from build123d import *
from build123d.topology import SkipClean

# Parameters (mm, degrees)
SKETCH_1_W          = 86
SKETCH_1_H          = 68
SKETCH_1_R          = 1.8
EXTRUDE_1_DEPTH     = 3
CUT_EXTRUDE_1_DEPTH = 3
SKETCH_3_W          = 30
SKETCH_3_H          = 6
SKETCH_3_R          = 1.6
EXTRUDE_2_DEPTH     = 3
EXTRUDE_3_DEPTH     = 3
SKETCH_5_R          = 1.5
CUT_EXTRUDE_2_DEPTH = 79.276480437
CUT_EXTRUDE_3_DEPTH = 79.276480437
EXTRUDE_4_DEPTH     = 3
EXTRUDE_6_DEPTH     = 3
CUT_EXTRUDE_6_DEPTH = 85.85098703
CUT_EXTRUDE_7_DEPTH = 85.85098703


with BuildPart() as part:
    # 草图1 → 凸台-拉伸1 (new body)
    with BuildSketch(Plane(origin=(0, 0, 0), x_dir=(1, 0, 0), z_dir=(0, 1, 0))):
        Rectangle(SKETCH_1_W, SKETCH_1_H)
        with Locations(Location((-36, -27, 0), (0, 0, 270))):
            Circle(SKETCH_1_R, mode=Mode.SUBTRACT)
        with Locations(Location((-36, 27, 0), (0, 0, 270))):
            Circle(SKETCH_1_R, mode=Mode.SUBTRACT)
        with Locations(Location((36, 27, 0), (0, 0, 270))):
            Circle(SKETCH_1_R, mode=Mode.SUBTRACT)
        with Locations(Location((36, -27, 0), (0, 0, 270))):
            Circle(SKETCH_1_R, mode=Mode.SUBTRACT)
    extrude(amount=EXTRUDE_1_DEPTH)

    # 草图2 → 切除-拉伸1 (cut)
    with BuildSketch(Plane.XZ):
        Polygon((26, 25), (35, 34), (-35, 34), (-26, 25), align=None)
        Polygon((-28, 13), (-43, 28), (-43, -28), (-28, -13), align=None)
        Polygon((-35, -34), (35, -34), (26, -25), (-26, -25), align=None)
        Polygon((43, -28), (43, 28), (28, 13), (28, -13), align=None)
    extrude(amount=-CUT_EXTRUDE_1_DEPTH, mode=Mode.SUBTRACT)

    # 草图3 → 凸台-拉伸2 (add)
    # profile 1 of 3: a face of its own
    with BuildSketch(Plane.XZ):
        Polygon((35, 34), (43, 34), (45.67228251, 57.499999999), (15.67228251, 57.499999999), (26, 25), align=None)
    # profile 2 of 3: a face of its own
    with BuildSketch(Plane.XZ):
        with Locations((30.67228251, 60.499999999)):
            Rectangle(SKETCH_3_W, SKETCH_3_H)
        with Locations(Location((20.67228251, 60.499999999, 0), (0, 0, 270))):
            Circle(SKETCH_3_R, mode=Mode.SUBTRACT)
        with Locations(Location((40.67228251, 60.499999999, 0), (0, 0, 270))):
            Circle(SKETCH_3_R, mode=Mode.SUBTRACT)
    # profile 3 of 3: a face of its own
    with BuildSketch(Plane.XZ):
        Polygon((45.67228251, -63.499999999), (45.67228251, -57.499999999), (43, -34), (35, -34), (26, -25), (15.67228251, -57.499999999), (15.67228251, -63.499999999), align=None)
        with Locations(Location((20.67228251, -60.499999999, 0), (0, 0, 270))):
            Circle(SKETCH_3_R, mode=Mode.SUBTRACT)
        with Locations(Location((40.67228251, -60.499999999, 0), (0, 0, 270))):
            Circle(SKETCH_3_R, mode=Mode.SUBTRACT)
    extrude(amount=-EXTRUDE_2_DEPTH)

    # 草图4 → 凸台-拉伸3 (add)
    with BuildSketch(Plane.XZ):
        Polygon((15.67228251, 57.499999999), (15.67228251, 63.499999999), (-43, 34), (-35, 34), align=None)
        Polygon((-35, -34), (-43, -34), (15.67228251, -63.499999999), (15.67228251, -57.499999999), align=None)
    extrude(amount=-EXTRUDE_3_DEPTH)

    # 草图5 → 切除-拉伸2 (cut, through all)
    with BuildSketch(Plane.XZ):
        with Locations(Location((-13.9, 10, 0), (0, 0, 270))):
            Circle(SKETCH_5_R)
        with Locations(Location((14.8, 10, 0), (0, 0, 270))):
            Circle(SKETCH_5_R)
        with Locations(Location((-13.9, -10, 0), (0, 0, 270))):
            Circle(SKETCH_5_R)
        with Locations(Location((14.8, -10, 0), (0, 0, 270))):
            Circle(SKETCH_5_R)
    extrude(amount=-CUT_EXTRUDE_2_DEPTH, mode=Mode.SUBTRACT)

    # 草图6 → 切除-拉伸3 (cut, through all)
    with BuildSketch(Plane.XZ):
        with BuildLine():
            Line((-21.292893219, 20.292893219), (-14.292893219, 13.292893219))
            ThreePointArc((-14.292893219, 13.292893219), (-13.96846987, 13.076120467), (-13.585786438, 13))
            Line((-13.585786438, 13), (13.485786438, 13))
            ThreePointArc((13.485786438, 13), (13.86846987, 13.076120467), (14.192893219, 13.292893219))
            Line((14.192893219, 13.292893219), (21.192893219, 20.292893219))
            ThreePointArc((21.192893219, 20.292893219), (21.40966597, 21.382683432), (20.485786438, 22))
            Line((20.485786438, 22), (-20.585786438, 22))
            ThreePointArc((-20.585786438, 22), (-21.50966597, 21.382683432), (-21.292893219, 20.292893219))
        make_face()
        with BuildLine():
            Line((-25, 7.585786438), (-25, -7.585786438))
            ThreePointArc((-25, -7.585786438), (-24.382683432, -8.50966597), (-23.292893219, -8.292893219))
            Line((-23.292893219, -8.292893219), (-17.192893219, -2.192893219))
            ThreePointArc((-17.192893219, -2.192893219), (-16.976120467, -1.86846987), (-16.9, -1.485786438))
            Line((-16.9, -1.485786438), (-16.9, 1.485786438))
            ThreePointArc((-16.9, 1.485786438), (-16.976120467, 1.86846987), (-17.192893219, 2.192893219))
            Line((-17.192893219, 2.192893219), (-23.292893219, 8.292893219))
            ThreePointArc((-23.292893219, 8.292893219), (-24.382683432, 8.50966597), (-25, 7.585786438))
        make_face()
        with BuildLine():
            Line((-9.9, 9), (9.9, 9))
            ThreePointArc((9.9, 9), (10.607106781, 8.707106781), (10.9, 8))
            Line((10.9, 8), (10.9, -8))
            ThreePointArc((10.9, -8), (10.607106781, -8.707106781), (9.9, -9))
            Line((9.9, -9), (-9.9, -9))
            ThreePointArc((-9.9, -9), (-10.607106781, -8.707106781), (-10.9, -8))
            Line((-10.9, -8), (-10.9, 8))
            ThreePointArc((-10.9, 8), (-10.607106781, 8.707106781), (-9.9, 9))
        make_face()
        with BuildLine():
            Line((14.192893219, -13.292893219), (21.192893219, -20.292893219))
            ThreePointArc((21.192893219, -20.292893219), (21.40966597, -21.382683432), (20.485786438, -22))
            Line((20.485786438, -22), (-20.585786438, -22))
            ThreePointArc((-20.585786438, -22), (-21.50966597, -21.382683432), (-21.292893219, -20.292893219))
            Line((-21.292893219, -20.292893219), (-14.292893219, -13.292893219))
            ThreePointArc((-14.292893219, -13.292893219), (-13.96846987, -13.076120467), (-13.585786438, -13))
            Line((-13.585786438, -13), (13.485786438, -13))
            ThreePointArc((13.485786438, -13), (13.86846987, -13.076120467), (14.192893219, -13.292893219))
        make_face()
        with BuildLine():
            Line((16.9, -1.485786438), (16.9, 1.485786438))
            ThreePointArc((16.9, 1.485786438), (16.976120467, 1.86846987), (17.192893219, 2.192893219))
            Line((17.192893219, 2.192893219), (23.292893219, 8.292893219))
            ThreePointArc((23.292893219, 8.292893219), (24.382683432, 8.50966597), (25, 7.585786438))
            Line((25, 7.585786438), (25, -7.585786438))
            ThreePointArc((25, -7.585786438), (24.382683432, -8.50966597), (23.292893219, -8.292893219))
            Line((23.292893219, -8.292893219), (17.192893219, -2.192893219))
            ThreePointArc((17.192893219, -2.192893219), (16.976120467, -1.86846987), (16.9, -1.485786438))
        make_face()
    extrude(amount=-CUT_EXTRUDE_3_DEPTH, mode=Mode.SUBTRACT)

    # 草图7 → 凸台-拉伸4 (add)
    with BuildSketch(Plane.XZ):
        Polygon((-56.2, 27.363135311), (-56.2, -27.363135311), (-43, -34), (-43, -28), (-52.2, -23.374306429), (-52.2, 23.374306429), (-43, 28), (-43, 34), align=None)
    extrude(amount=-EXTRUDE_4_DEPTH)

    # 草图11 → 凸台-拉伸6 (add)
    with BuildSketch(Plane.XZ):
        with BuildLine():
            Line((35.3, 1.5), (35.3, 18.5))
            ThreePointArc((35.3, 18.5), (34.629179607, 18.658359214), (34.1, 19.1))
            Line((34.1, 19.1), (28, 13))
            Line((28, 13), (28, -13))
            Line((28, -13), (34.1, -19.1))
            ThreePointArc((34.1, -19.1), (34.629179607, -18.658359214), (35.3, -18.5))
            Line((35.3, -18.5), (35.3, -1.5))
            ThreePointArc((35.3, -1.5), (33.8, 0), (35.3, 1.5))
        make_face()
        with BuildLine():
            ThreePointArc((36.8, 20), (36.360660172, 18.939339828), (35.3, 18.5))
            Line((35.3, 18.5), (35.3, 1.5))
            ThreePointArc((35.3, 1.5), (36.360660172, 1.060660172), (36.8, 0))
            ThreePointArc((36.8, 0), (36.360660172, -1.060660172), (35.3, -1.5))
            Line((35.3, -1.5), (35.3, -18.5))
            ThreePointArc((35.3, -18.5), (36.360660172, -18.939339828), (36.8, -20))
            ThreePointArc((36.8, -20), (36.641640786, -20.670820393), (36.2, -21.2))
            Line((36.2, -21.2), (38.3, -23.3))
            Line((38.3, -23.3), (38.3, 23.3))
            Line((38.3, 23.3), (36.2, 21.2))
            ThreePointArc((36.2, 21.2), (36.641640786, 20.670820393), (36.8, 20))
        make_face()
    extrude(amount=-EXTRUDE_6_DEPTH)

    # 草图11<3> → 切除-拉伸6 (cut, through all)
    with SkipClean():  # the faces are left unmerged after this step: merging them gives an invalid solid
        with BuildSketch(Plane.XZ):
            with BuildLine():
                ThreePointArc((36.2, 21.2), (34.239339828, 21.060660172), (34.1, 19.1))
                Line((34.1, 19.1), (36.2, 21.2))
            make_face()
            with BuildLine():
                Line((36.2, 21.2), (34.1, 19.1))
                ThreePointArc((34.1, 19.1), (35.774341649, 18.576975053), (36.8, 20))
                ThreePointArc((36.8, 20), (36.641640786, 20.670820393), (36.2, 21.2))
            make_face()
            with BuildLine():
                ThreePointArc((36.8, -20), (35.774341649, -18.576975053), (34.1, -19.1))
                Line((34.1, -19.1), (36.2, -21.2))
                ThreePointArc((36.2, -21.2), (36.641640786, -20.670820393), (36.8, -20))
            make_face()
            with BuildLine():
                Line((36.2, -21.2), (34.1, -19.1))
                ThreePointArc((34.1, -19.1), (34.239339828, -21.060660172), (36.2, -21.2))
            make_face()
        extrude(amount=-CUT_EXTRUDE_6_DEPTH, mode=Mode.SUBTRACT)

    # 草图12 → 切除-拉伸7 (cut, through all)
    with SkipClean():  # the faces are left unmerged after this step: merging them gives an invalid solid
        with BuildSketch(Plane.XZ):
            with BuildLine():
                Line((21.125963718, 53.545721451), (27.85115527, 32.382407713))
                ThreePointArc((27.85115527, 32.382407713), (29.426324108, 31.343770669), (30.771106367, 32.667207276))
                Line((30.771106367, 32.667207276), (33.177674586, 53.830521014))
                ThreePointArc((33.177674586, 53.830521014), (32.806256586, 54.998944823), (31.687279714, 55.499999999))
                Line((31.687279714, 55.499999999), (22.555519943, 55.499999999))
                ThreePointArc((22.555519943, 55.499999999), (21.344855286, 54.885602104), (21.125963718, 53.545721451))
            make_face()
            with BuildLine():
                Line((30.771106367, -32.667207276), (33.177674586, -53.830521014))
                ThreePointArc((33.177674586, -53.830521014), (32.806256586, -54.998944823), (31.687279714, -55.499999999))
                Line((31.687279714, -55.499999999), (22.555519943, -55.499999999))
                ThreePointArc((22.555519943, -55.499999999), (21.344855286, -54.885602104), (21.125963718, -53.545721451))
                Line((21.125963718, -53.545721451), (27.85115527, -32.382407713))
                ThreePointArc((27.85115527, -32.382407713), (29.426324108, -31.343770669), (30.771106367, -32.667207276))
            make_face()
        extrude(amount=-CUT_EXTRUDE_7_DEPTH, mode=Mode.SUBTRACT)


solid = part.part
Read the model definition and answer for the solid it produces. Units are mm, in the model's axes. Give positions to 0.01 mm unless a question says otherwise; leave off trailing zeros. Write each loop counter-clockwise with the first axis right and the second up, starting at its lowest first coordinate (ties: lowest second). Pieces come first, ordered by that corner, then holes. Notation, with made-up numbers: M -37.5,39.25 L 10.5,39.25 A18 cw 10.5,53.25 Z; hole C -8.5,78 d1. An arc over 180 degrees is marked long. One line per item, written item: value. Start each with the question number.
(1) Determine the mould class of faces 1 (the cylindrical face through (13.336, 1.479, 10.325)), 2 (the flat face through (41, 1, -26)), 3 (the flat face through (-56.2, 1, 0)) for opening direction X: pulls with the +X half, pulls with the -X half, needs draft (parallel to the pull), parting line crosses it, or undercut.
(2) Find the intervals of material crossed by line 1 (X direction, y = 1.05, z = 7); line 2 (X direction, y = 0.6, z = 10); line 3 (Z direction, x = 40, y = 0.75), in increasing order.
(3) Find section B-B (z = 38). Determine the outline of the cut face in (x, y), plus the area to 3 significant figures.
(4) Flat-ended cylindrical pins translate along their axes: pin 1 Ø1.5 at (y, z) = (1, -30) entering from +X; pin 2 Ø1.5 at (y, z) = (1, 1.5) entering from +X. Find the tip coordinate at first contact, or state that the pin passes through.
(5) Find section A-A (x = -2.5). Determine the outline of the cut face in (y, z).
(6) Find section C-C (y = 1.8). Give the number of separate pieces and of enclosed holes in the cut face, plus the area to 3 significant figures.
Results below:
1. face 1: undercut
1. face 2: pulls with the +X half
1. face 3: pulls with the -X half
2. line 1: x = -56.2 to -52.2, -28 to -25, -22 to -10.9, 10.9 to 22, 25 to 38.3
2. line 2: x = -56.2 to -52.2, -28 to -15.4, -12.4 to 13.3, 16.3 to 38.3
2. line 3: z = -63.5 to -61.95, -59.05 to -25, 25 to 59.05, 61.95 to 63.5
3. outline: M -35.04,0 L -26.37,0 L -26.37,3 L -35.04,3 Z; M 21.87,0 L 26.07,0 L 26.07,3 L 21.87,3 Z; M 31.38,0 L 43.45,0 L 43.45,3 L 31.38,3 Z
3. area: 74.8 mm^2
4. pin 1: stops at x = 43
4. pin 2: stops at x = 38.3
5. outline: M 0,-54.36 L 3,-54.36 L 3,-49.07 L 0,-49.07 Z; M 0,-25 L 3,-25 L 3,-22 L 0,-22 Z; M 0,-13 L 3,-13 L 3,-9 L 0,-9 Z; M 0,9 L 3,9 L 3,13 L 0,13 Z; M 0,22 L 3,22 L 3,25 L 0,25 Z; M 0,49.07 L 3,49.07 L 3,54.36 L 0,54.36 Z
6. separate pieces: 1
6. enclosed holes: 25
6. area: 4,680 mm^2
